from build123d import *

# Parameters (mm, degrees)
F1_DEPTH      = 46.228
F2_R          = 7.092967
F3_DEPTH      = 5.08
F3_DEPTH_BACK = 5.08


with BuildPart() as f1:
    # F0 (on Front) → F1 (new body)
    with BuildSketch(Plane.XZ):
        Polygon((-53.001549, 10.965838), (-62.545888, 0), (67.419596, 0), (64.779676, 15.027259), (45.690991, 16.854899), (34.928225, 27.008452), (5.076777, 28.836092), (-18.479466, 15.636472), align=None)
    extrude(amount=F1_DEPTH)

    # F2 (on face) → F3 (join, two sides)
    with BuildSketch(Plane.XZ.offset(46.228)) as f3_sk:
        with Locations((-39.395787, -2.030711)):
            Circle(F2_R)
    extrude(amount=F3_DEPTH)
    extrude(f3_sk.sketch, amount=-F3_DEPTH_BACK)


solid = f1.part
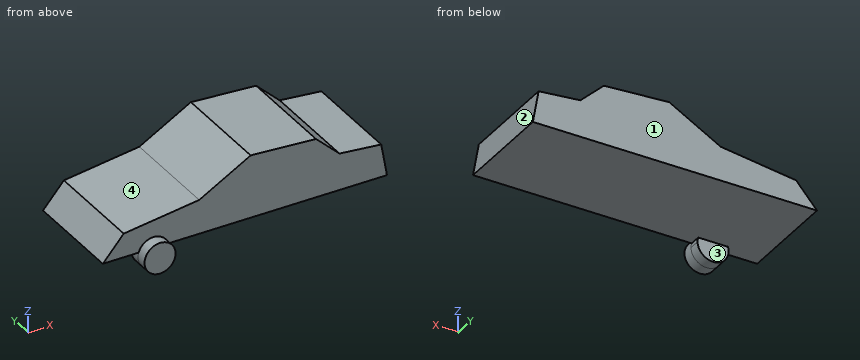
The model under review builds one solid part; all positions refer to its coordinate system, in mm. Face numbers are marked on the shaded views. A direction names the side the tool comes from. Round coordinates to 2 decimals unless told otherwise and drop trailing zeros. Write each loop counter-clockwise with the first axis right and the second up, starting at its lowest first coordinate (ties: lowest second). Pieces come first, ordered by that corner, then holes. Notation, with made-up numbers: (65, 87.25) - (101, 87.25) arc R10 cw to (101, 96.25) - close; hole circle Ø8 at (29.5, 28). An arc over 180 degrees is marked (long way). One line per item, written item: value. Start each with the question number.
1. Consider section C-C on z = 18.5. Write out the cut boundary in (x, y), and give its area (3 significant figures).
2. To check wall thickness, follow L1, parallel to Y at x = -54, z = 0.5; L2, parallel to Y at x = -33, z = -4; L3, parallel to X at y = -26, z = 20. State the ranges of each line that lie inside material, in increasing order. Write a range as from..to.
3. Machinability: for the marked faces 3 and 4, which of the approach directions +Z, -Z, +X, -X, +Y, -Y give a long, thin tool a straight path to every point of the face, cutting with its end or side? Answer none if there is none.
4. Consider section B-B on x = -0.5. Write out the cut boundary in (y, z), and give its area (3 significant figures).
5. Clearance check with flat-ended pins moving along their axes: P1, Ø14, axis at x = 30.5, y = -23, coming from the -Z side; P2, Ø6, axis at x = 18.5, z = 2.5, coming from the -Y side; P3, Ø7.5, axis at x = -39, z = -5, coming from the +Y side. State where each tip first meets the part, or that it passes through.
6. Consider section A-A on y = -38. Write out the cut boundary in (x, z), and give its area (3 significant figures).
7. The part is to be moulded in two halves that separate along Z. For the marked faces 1 and 2, say which applies: released by +Z, released by -Z, zero draft, split by the parting line, or undercut.
Checks:
1. outline: (-13.37, -46.23) - (43.95, -46.23) - (43.95, 0) - (-13.37, 0) - close
1. area: 2,650 mm^2
2. L1: y = -46.23..0
2. L2: y = -51.31..-41.15
2. L3: x = -10.69..42.36
3. face 3: -Z, +X, -X, +Y
3. face 4: +Z, -X, +Y, -Y
4. outline: (-46.23, 0) - (0, 0) - (0, 25.71) - (-46.23, 25.71) - close
4. area: 1,190 mm^2
5. P1: stops at z = 0
5. P2: stops at y = -46.23
5. P3: stops at y = -41.15
6. outline: (-62.55, 0) - (67.42, 0) - (64.78, 15.03) - (45.69, 16.85) - (34.93, 27.01) - (5.08, 28.84) - (-18.48, 15.64) - (-53, 10.97) - close
6. area: 2,430 mm^2
7. face 1: zero draft
7. face 2: released by +Z
